from build123d import *

# Parameters (mm, degrees)
F0_R     = 27.051
F1_DEPTH = 3.175
F4_D     = 2.9464
F5_D     = 2.1844
F7_D     = 8.382


with BuildPart() as f1:
    # F0 (on Top) → F1 (new body)
    with BuildSketch(Plane.XY):
        Circle(F0_R)
    extrude(amount=F1_DEPTH)

    # F4 (through all)
    with Locations(Plane.XY.offset(3.175)):
        with Locations((12.573, 21.7678), (21.7678, 12.573), (21.7678, -12.573), (12.573, -21.7678), (-12.573, -21.7678), (-12.573, 21.7678), (-21.7678, 12.573), (-21.7678, -12.573)):
            Hole(F4_D / 2)

    # F5 (through all)
    with Locations(Plane.XY.offset(3.175)):
        with Locations((8.128, -4.699), (8.1389067448, 4.699), (0.0054533724, 9.388554482), (-8.1389067448, 4.699), (-8.1334533724, -4.689554482), (0, -9.398)):
            Hole(F5_D / 2)

    # F7 (through all)
    with Locations(Plane.XY.offset(3.175)):
        with Locations((0, 0)):
            Hole(F7_D / 2)


solid = f1.part
Design review of the part built by this model. Coordinates are the model's own, in mm. Give positions to 0.01 mm unless a question says otherwise; leave off trailing zeros. Loops run counter-clockwise (first coordinate to the right, second up) from the corner with the lowest first, then second, coordinate; pieces in that order, holes last. Notation, with made-up numbers: M 0,63 L 23,63 A15 ccw 23,81 Z; hole C 3.25,20 d11. An arc over 180 degrees is marked long. One line per question, with ' | ' between items. Start each with the question number.
1. Add section A-A (y = 0). Write out the cut boundary in (x, z) (3 decimals).
2. Add section B-B (x = 0). Write out the cut boundary in (y, z) (3 decimals).
3. Insertion check: P1, Ø1.8, axis at x = 12.57, y = 21.77, coming from the -Z side; P2, Ø1, axis at x = -8.5, z = 2, coming from the -Y side; P3, Ø1, axis at x = 1, z = 2, coming from the -Y side. Each pin has a flat end and moves straight along its axis. Give the tip position at first contact, or say it passes through.
4. To check wall thickness, follow L1, parallel to Y at x = -12.5, z = 0.4; L2, parallel to X at y = 10, z = 2.3; L3, parallel to Y at x = -21.5, z = 2.35. State the ranges of each line that lie inside material, in increasing order.
5. Add section D-D (x = 22). Write out the cut boundary in (y, z) (3 decimals).
6. Add section C-C (z = 1.9). Give the number of separate pieces and of enclosed holes in the cut face, plus the area to 3 significant figures.
Worked out:
1) outline: M -27.051,0 L -4.191,0 L -4.191,3.175 L -27.051,3.175 Z; M 4.191,0 L 27.051,0 L 27.051,3.175 L 4.191,3.175 Z
2) outline: M -27.051,0 L -10.49,0 L -10.49,3.175 L -27.051,3.175 Z; M -8.306,0 L -4.191,0 L -4.191,3.175 L -8.306,3.175 Z; M 4.191,0 L 8.296,0 L 8.296,3.175 L 4.191,3.175 Z; M 10.481,0 L 27.051,0 L 27.051,3.175 L 10.481,3.175 Z
3) P1: passes through | P2: stops at y = -25.84 | P3: stops at y = -27.05
4) L1: y = -23.99 to -23.24, -20.3 to 20.3, 23.24 to 23.99 | L2: x = -25.13 to -0.9, 0.91 to 25.13 | L3: y = -16.42 to -14.02, -11.12 to 11.12, 14.02 to 16.42
5) outline: M -15.74,0 L -14.028,0 L -14.028,3.175 L -15.74,3.175 Z; M -11.118,0 L 11.118,0 L 11.118,3.175 L -11.118,3.175 Z; M 14.028,0 L 15.74,0 L 15.74,3.175 L 14.028,3.175 Z
6) separate pieces: 1 | enclosed holes: 15 | area: 2,170 mm²
